Check sheet for the drawn part. Datum: minimum x, y, z corner. Units: mm. A direction names the side the tool comes from. Give positions to 0.01 mm unless a question says otherwise; leave off trailing zeros. Write each loop counter-clockwise with the first axis right and the second up, starting at its lowest first coordinate (ties: lowest second). Pieces come first, ordered by that corner, then holes.
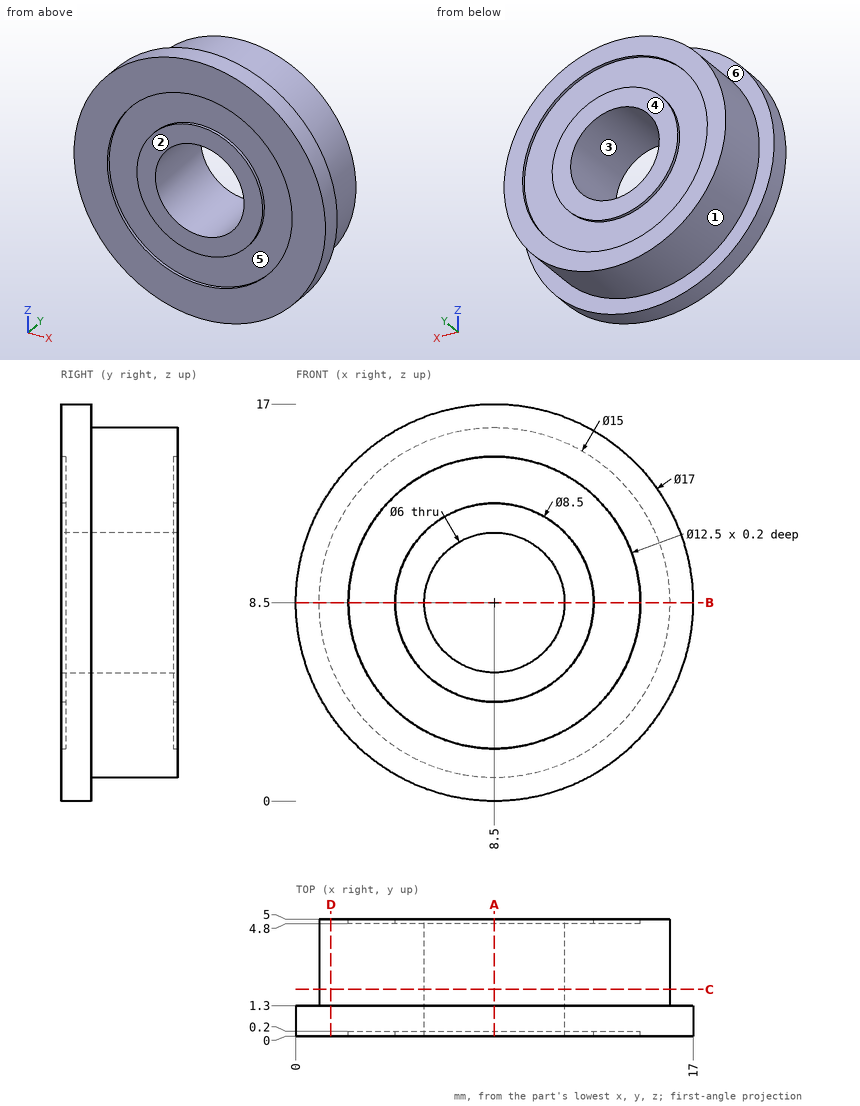
1) Sectioned sample at B-B on z = 8.5. Record the boundary of the cut face in (x, y).
2) Access from +Z, -Z, +X, -X, +Y, -Y to the whole of each face (thin tool, end or side, straight path). Record for the marked faces 4, 5 and 6.
3) Gauge pin test, flat ends, axial feed: pin 1 (3 mm diameter, centred on y = 3.5, z = 11, fed in from -X); pin 2 (5.5 mm diameter, centred on x = 8.5, z = 8.5, fed in from +Y); pin 3 (4 mm diameter, centred on x = 10.5, z = 9.5, fed in from -Y). Record the tip position at first contact, or that the pin passes through.
4) Scan lines: L1, parallel to X at y = 0.1, z = 8.5; L2, parallel to X at y = 3.15, z = 8.5; L3, parallel to Y at x = 11.25, z = 1.25. Record each from-to range of solid material in increasing order.
5) Sectioned sample at D-D on x = 1.5. Record the boundary of the cut face in (y, z), then the cut area to 3 significant figures.
6) Draft check along Z on the marked faces 1, 2 and 3. Enter one of: +Z half, -Z half, draft (parallel to the pull), parting line (faces both ways), or undercut.
7) Sectioned sample at C-C on y = 2. Record the boundary of the cut face in (x, z), then the cut area to 3 significant figures.
8) Sectioned sample at A-A on x = 8.5. Record the boundary of the cut face in (y, z).
Answers below:
1. outline: (0, 0) - (2.25, 0) - (2.25, 0.2) - (4.25, 0.2) - (4.25, 0) - (5.5, 0) - (5.5, 5) - (4.25, 5) - (4.25, 4.8) - (2.25, 4.8) - (2.25, 5) - (1, 5) - (1, 1.3) - (0, 1.3) - close; (11.5, 0) - (12.75, 0) - (12.75, 0.2) - (14.75, 0.2) - (14.75, 0) - (17, 0) - (17, 1.3) - (16, 1.3) - (16, 5) - (14.75, 5) - (14.75, 4.8) - (12.75, 4.8) - (12.75, 5) - (11.5, 5) - close
2. face 4: +Z, -Z, +X, -X, +Y
2. face 5: -Y
2. face 6: +Y
3. pin 1: stops at x = 1.07
3. pin 2: passes through
3. pin 3: stops at y = 0
4. L1: x = 0 to 2.25, 4.25 to 5.5, 11.5 to 12.75, 14.75 to 17
4. L2: x = 1 to 5.5, 11.5 to 16
4. L3: y = 0 to 1.3
5. outline: (0, 3.68) - (1.3, 3.68) - (1.3, 5.81) - (5, 5.81) - (5, 11.19) - (1.3, 11.19) - (1.3, 13.32) - (0, 13.32) - close
5. area: 32.5 mm2
6. face 1: parting line
6. face 2: draft
6. face 3: undercut
7. outline: circle Ø15 at (8.5, 8.5); hole circle Ø6 at (8.5, 8.5)
7. area: 148 mm2
8. outline: (0, 0) - (1.3, 0) - (1.3, 1) - (5, 1) - (5, 2.25) - (4.8, 2.25) - (4.8, 4.25) - (5, 4.25) - (5, 5.5) - (0, 5.5) - (0, 4.25) - (0.2, 4.25) - (0.2, 2.25) - (0, 2.25) - close; (0, 11.5) - (5, 11.5) - (5, 12.75) - (4.8, 12.75) - (4.8, 14.75) - (5, 14.75) - (5, 16) - (1.3, 16) - (1.3, 17) - (0, 17) - (0, 14.75) - (0.2, 14.75) - (0.2, 12.75) - (0, 12.75) - close
